Autodesk Inventor part; units mm, degrees
ref_plane "YZ Plane" through (0, 0, 0) normal (1, 0, 0) x (0, 1, 0)
ref_plane "XZ Plane" through (0, 0, 0) normal (0, 1, 0) x (-1, 0, 0)
ref_plane "XY Plane" through (0, 0, 0) normal (0, 0, 1) x (1, 0, 0)
sketch "Sketch1" plane through (0, 0, 0) normal (0, 0, 1) x (1, 0, 0)
  line L0 (13.75, -11) -> (-13.75, -11)
  line L1 (-13.75, -11) -> (-13.75, 11)
  line L2 (-13.75, 11) -> (13.75, 11)
  line L3 (13.75, 11) -> (13.75, -11)
  line L4 (13.75, -11) -> (-13.75, 11) construction
  line L5 (-13.75, -11) -> (13.75, 11) construction
  circle A0 centre (0, 0) radius 5.4
  dimension "d0" = 27.5
  dimension "d1" = 22
  dimension "d2" = 10.8
extrude "Extrusion1" add sketch "Sketch1" along normal blind 1
sketch "Sketch2" plane through (0, 0, 0) normal (0, 0, -1) x (-1, 0, 0)
  line L0 (15.25, 12.5) -> (-15.25, 12.5)
  line L1 (-15.25, 12.5) -> (-15.25, -12.5)
  line L2 (-15.25, -12.5) -> (15.25, -12.5)
  line L3 (15.25, -12.5) -> (15.25, 12.5)
  line L4 (15.25, 12.5) -> (-15.25, -12.5) construction
  line L5 (-15.25, 12.5) -> (15.25, -12.5) construction
  line L6 (-13.75, -11) -> (-13.75, 11)
  line L7 (-13.75, 11) -> (13.75, 11)
  circle A0 centre (0, 0) radius 5.4
  circle A1 centre (0, 0) radius 5.4
  dimension "d5" = 1.5
  dimension "d6" = 1.5
extrude "Extrusion2" add sketch "Sketch2" along normal blind 1
fillet "Fillet1" radius 3 4 edges at (-15.25, 12.5, -0.5) (-15.25, -12.5, -0.5) (15.25, -12.5, -0.5) (15.25, 12.5, -0.5)
properties part number "screen-dc-port-front"
For this review, take the finished solid that the model builds, in its own axes (mm). A direction names the side the tool comes from. Round coordinates to 2 decimals unless told otherwise and drop trailing zeros. Write each loop counter-clockwise with the first axis right and the second up, starting at its lowest first coordinate (ties: lowest second). Pieces come first, ordered by that corner, then holes.
1) Insertion check: pin 1 Ø0.8 at (x, z) = (6, 0.5) entering from +Y; pin 2 Ø0.8 at (y, z) = (-2.5, 0.5) entering from -X; pin 3 Ø0.8 at (y, z) = (0.5, 0.5) entering from +X. Each pin has a flat end and moves straight along its axis. Give the tip position at first contact, or say it passes through.
Answer below:
pin 1: stops at y = 11
pin 2: stops at x = -13.75
pin 3: stops at x = 13.75
2) Take a section at D-D on y = -8.25. Give the boundary of the cut face in (x, z).
Answer below:
outline: (-15.25, -1) - (15.25, -1) - (15.25, 0) - (13.75, 0) - (13.75, 1) - (-13.75, 1) - (-13.75, 0) - (-15.25, 0) - close
3) Take a section at C-C on z = 0.45. Give the boundary of the cut face in (x, y).
Answer below:
outline: (-13.75, -11) - (13.75, -11) - (13.75, 11) - (-13.75, 11) - close; hole circle Ø10.8 at (0, 0)
4) Take a section at A-A on y = 0. Give the boundary of the cut face in (x, z).
Answer below:
outline: (-15.25, -1) - (-5.4, -1) - (-5.4, 1) - (-13.75, 1) - (-13.75, 0) - (-15.25, 0) - close; (5.4, -1) - (15.25, -1) - (15.25, 0) - (13.75, 0) - (13.75, 1) - (5.4, 1) - close
5) For line 1 along Y through (x, z) = (0, -0.3); line 2 along X through (y, z) = (0, -0.3); line 3 along Y through (x, z) = (0, 0.6), list the stretches that pass through material, from the lowest coordinate up.
Answer below:
line 1: y = -12.5 to -5.4, 5.4 to 12.5
line 2: x = -15.25 to -5.4, 5.4 to 15.25
line 3: y = -11 to -5.4, 5.4 to 11
6) Machinability: for faces 1 (the face through (-13.75, -0.2, 0.5)), 2 (the face through (0.2, -11, 0.5)), 3 (the face through (13.75, 0.2, 0.5)), 4 (the face through (-0.2, 11, 0.5)), which of the approach directions +Z, -Z, +X, -X, +Y, -Y give a long, thin tool a straight path to every point of the face, cutting with its end or side? Answer none if there is none.
Answer below:
face 1: +Z, -X, +Y, -Y
face 2: +Z, +X, -X, -Y
face 3: +Z, +X, +Y, -Y
face 4: +Z, +X, -X, +Y
7) Take a section at B-B on x = 0. Give the boundary of the cut face in (y, z).
Answer below:
outline: (-12.5, -1) - (-5.4, -1) - (-5.4, 1) - (-11, 1) - (-11, 0) - (-12.5, 0) - close; (5.4, -1) - (12.5, -1) - (12.5, 0) - (11, 0) - (11, 1) - (5.4, 1) - close
